Solid Edge part; units mm, degrees
sketch "Sketch1" plane through (0, 0, 0) normal (1, 0, 0) x (0, 1, 0)
  line L0 (-40.6829, -217.8929) -> (-40.6829, 12.1071)
  line L1 (-40.6829, 12.1071) -> (-70.6829, 12.1071)
  line L2 (-70.6829, 12.1071) -> (-70.6829, -217.8929)
  line L3 (-70.6829, -217.8929) -> (-40.6829, -235.2134)
  line L4 (-40.6829, -235.2134) -> (-40.6829, -217.8929)
  line L5 (-70.6829, 12.1071) -> (-40.6829, 12.1071)
  line L6 (-54.1753, 28.1984) -> (-40.6829, 12.1071)
  line L7 (-57.1901, 28.1988) -> (-54.1753, 28.1984)
  line L8 (-70.6829, 12.1071) -> (-57.1901, 28.1988)
  dimension "D1" = 70.6829
  dimension "D2" = 54.1753
  dimension "D3" = 70.6829
  dimension "D4" = 40.6829
  dimension "D5" = 40.6829
  dimension "D6" = 0
extrude "Protrusion1" add sketch "Sketch1" against normal blind 3
sketch "Sketch2" plane through (0, -21.8205, 20.1807) normal (1, 0, 0) x (0, 1, 0)
  circle A0 centre (-33.8622, -156.9821) radius 5
  circle A1 centre (-33.8621, -1.9821) radius 5
extrude "ExtrudedProtrusion_2" add sketch "Sketch2" along normal blind 11
mirror "Mirror1" about plane through (5, -21.8205, 20.1506) normal (1, 0, 0) of "Protrusion1"
sketch "Sketch3" plane through (-1.5, -55.6829, -226.5532) normal (0, -0.5, -0.866) x (0, -0.866, 0.5)
  circle A0 centre (0, -6.5) radius 50
extrude "ExtrudedProtrusion_5" add sketch "Sketch3" along normal blind 5
sketch "Sketch4" plane through (5, -58.1829, -230.8833) normal (0, -0.5, -0.866) x (-1, 0, 0)
  circle A0 centre (0, 0) radius 20
extrude "ExtrudedProtrusion_6" add sketch "Sketch4" along normal blind 10
Input: part model. Units: mm. Frame: model coordinates. A direction names the side the tool comes from. Give positions to 0.01 mm unless a question says otherwise; leave off trailing zeros. Write each loop counter-clockwise with the first axis right and the second up, starting at its lowest first coordinate (ties: lowest second). Pieces come first, ordered by that corner, then holes.
Q1. Pull-direction query (Z, two-part tool) for faces 1 (the face through (20, -98.2, -204.8)), 2 (the face through (13, -56, -102)), 3 (the face through (-13.475, -54.014, -238.983)); classes: pulls with the +Z half, pulls with the -Z half, needs draft (parallel to the pull), parting line crosses it, or undercut.
Q2. Section A-A, the plane z = -72.5. Output: boundary loops of the cut face in (x, y), plus the area to 3 significant figures.
Q3. Set-up query: faces 4 (the face through (4.93, -59.65, 21.24)), 5 (the face through (11.48, -63.84, 20.27)). Return all of +Z, -Z, +X, -X, +Y, -Y with unobstructed straight access to the full face (end or side cutting, diameter ignored); none if empty.
Q4. First-contact query: P1, Ø12, axis at x = -3, y = -77.5, coming from the +Z side; P2, Ø9, axis at y = -58, z = -121.5, coming from the +X side; P3, Ø2.5, axis at x = 11.5, z = -152, coming from the -Y side. Flat tips, straight axial feed; report the tip coordinate or a pass-through.
Q5. Section C-C, the plane x = -20. Output: boundary loops of the cut face in (y, z).
Q6. Section B-B, the plane x = 40.5. Output: boundary loops of the cut face in (y, z).
Q7. Material intervals for probe 1 along X at (y, z) = (-46, -188.5); probe 2 along Z at (x, y) = (-14, -80); probe 3 along Z at (x, y) = (15, -78.5), sorted ascending.
Filled in:
1. face 1: parting line crosses it
1. face 2: needs draft
1. face 3: undercut
2. outline: (-3, -70.68) - (0, -70.68) - (0, -40.68) - (-3, -40.68) - close; (10, -70.68) - (13, -70.68) - (13, -40.68) - (10, -40.68) - close
2. area: 180 mm2
3. face 4: none
3. face 5: +Z, +X, -X, -Y
4. P1: stops at z = -210.49
4. P2: stops at x = 13
4. P3: stops at y = -70.68
5. outline: (-95.68, -209.23) - (-20.68, -252.53) - (-18.18, -248.2) - (-93.18, -204.9) - close
6. outline: (-88.68, -213.28) - (-27.69, -248.49) - (-25.19, -244.16) - (-86.18, -208.95) - close
7. probe 1: x = -3 to 0, 10 to 13
7. probe 2: z = -218.29 to -212.51
7. probe 3: z = -219.15 to -213.38
